Autodesk Inventor part; units mm, degrees
ref_plane "YZ Plane" through (0, 0, 0) normal (1, 0, 0) x (0, 1, 0)
ref_plane "XZ Plane" through (0, 0, 0) normal (0, 1, 0) x (-1, 0, 0)
ref_plane "XY Plane" through (0, 0, 0) normal (0, 0, 1) x (1, 0, 0)
sketch "Sketch1" plane through (0, 0, 0) normal (1, 0, 0) x (0, 1, 0)
  line L0 (112.7241, 89.8734) -> (-26.9759, 89.8734)
  line L1 (-26.9759, 89.8734) -> (-26.9759, -24.4266)
  line L2 (-26.9759, -24.4266) -> (112.7241, -24.4266)
  line L3 (112.7241, -24.4266) -> (112.7241, 89.8734)
  point P0 (0, 0)
  dimension "d0" = 114.3
  dimension "d1" = 139.7
extrude "Extrusion1" add sketch "Sketch1" along normal blind 127
sketch "Sketch2" plane through (0, 112.7241, 89.8734) normal (0, 1, 0) x (1, 0, 0)
  line L0 (0, 0) -> (127, 0)
  line L1 (0, 114.3) -> (127, 114.3)
  line L2 (25.4, 0) -> (127, 0)
  line L3 (127, 0) -> (127, 114.3)
  line L4 (127, 114.3) -> (25.4, 114.3)
  line L5 (25.4, 114.3) -> (25.4, 0)
  line L6 (0, 114.3) -> (0, 0)
  point P0 (0, 89.8734)
  dimension "d4" = 25.4
extrude "Extrusion2" cut sketch "Sketch2" against normal blind 25.4 contours L5 L1 L3 L0
sketch "Sketch4" plane through (0, 87.3241, 89.8734) normal (0, 1, 0) x (1, 0, 0)
  line L0 (38.1, 127) -> (38.1, 0)
  circle A0 centre (76.2, 57.15) radius 44.45
  line L1 (127, 114.3) -> (127, 0)
  line L2 (127, 0) -> (25.4, 0)
  point P0 (0, 89.8734)
  dimension "d15" = 50.8
  dimension "d16" = 57.15
  dimension "d54" = 88.9
extrude "Extrusion4" cut sketch "Sketch4" against normal blind 63.5
fillet "Fillet3" radius 38.1 1 edges at (127, 30.1741, 89.8734)
fillet "Fillet4" radius 38.1 1 edges at (127, 30.1741, -24.4266)
sketch "Sketch9" plane through (25.4, 112.7241, 89.8734) normal (1, 0, 0) x (0, 0, -1)
  line L0 (0, 0) -> (114.3, 0)
  line L1 (0, -25.4) -> (0, 0)
  point P0 (89.8734, -112.7241)
  point P1 (57.15, -12.7)
  dimension "d30" = 12.7
  dimension "d31" = 57.15
hole "Hole1" at (25.4, 100.0241, 32.7234) direction (-1, 0, 0) diameter 8.4328 end through all counterbore diameter 20.6502 counterbore depth 5.969
sketch "Sketch10" plane through (0, -26.9759, -24.4266) normal (0, -1, 0) x (1, 0, 0)
  line L0 (0, 114.3) -> (88.9, 114.3)
  line L1 (25.4, 114.3) -> (127, 114.3)
  line L2 (127, 114.3) -> (127, 0)
  line L3 (127, 0) -> (25.4, 0)
  line L4 (25.4, 0) -> (25.4, 114.3)
  line L5 (0, 114.3) -> (0, 0)
  point P0 (0, 24.4266)
  dimension "d39" = 25.4
  dimension "d42" = 114.3
  dimension "d60" = 101.6
extrude "Extrusion6" cut sketch "Sketch10" against normal blind 25.4
sketch "Sketch11" plane through (25.4, -26.9759, 89.8734) normal (1, 0, 0) x (0, 0, -1)
  line L0 (114.3, 0) -> (0, 0)
  line L1 (114.3, 25.4) -> (114.3, 0)
  point P0 (89.8734, 26.9759)
  point P1 (57.15, 12.7)
  dimension "d43" = 12.7
  dimension "d44" = 57.15
hole "Hole2" at (25.4, -14.2759, 32.7234) direction (-1, 0, 0) diameter 8.4328 end through all counterbore diameter 20.6502 counterbore depth 5.969
sketch "Sketch15" plane through (0, -26.9759, -24.4266) normal (0, 0, -1) x (-1, 0, 0)
  line L0 (-25.4, 114.3) -> (-88.9, 114.3)
  line L1 (-76.2, 114.3) -> (-69.85, 114.3)
  line L2 (-69.85, 114.3) -> (-69.85, 50.8)
  line L3 (-69.85, 50.8) -> (-76.2, 50.8)
  line L4 (-76.2, 50.8) -> (-76.2, 114.3)
  line L5 (-127, 114.3) -> (-127, 0)
  point P0 (0, 26.9759)
  point P1 (-127, 25.4)
  dimension "d55" = 6.35
  dimension "d56" = 50.8
  dimension "d57" = 63.5
extrude "Extrusion8" cut sketch "Sketch15" against normal blind 25.4
properties part number "Cleaning Bottle Holder"
Work out the finished part from the listing and answer in its coordinate system (mm). A direction names the side the tool comes from. Round coordinates to 2 decimals unless told otherwise and drop trailing zeros. Order: outer loops, then holes, each group sorted by start corner. A loop starts at its lowest first (then second) coordinate and runs counter-clockwise, first axis right, second up. Notation, with made-up numbers: M -20,78 L -2,78 A31 ccw -2,109 Z; hole C -4.75,-34 d7. An arc over 180 degrees is marked long. One line per item, written item: value.
Q1. Find section D-D on y = 7. Write down the section's boundary in (x, z), then the cut area to 3 significant figures.
Derived:
outline: M 0,-24.43 L 88.9,-24.43 A38.1 ccw 127,13.67 L 127,51.77 A38.1 ccw 88.9,89.87 L 0,89.87 Z
area: 13,900 mm²
Q2. Determine the mould class of faces 1 (the face through (9.579, 99.839, 36.936)), 2 (the face through (25.4, 89, 32)), 3 (the face through (19.431, -9.8, 32.9)), 4 (the face through (30, 87.324, 32)) for opening direction Y: released by +Y, released by -Y, zero draft, split by the parting line, or undercut.
Derived:
face 1: undercut
face 2: zero draft
face 3: undercut
face 4: released by +Y
Q3. Flat-ended cylindrical pins translate along their axes: pin 1 (14.5 mm diameter, centred on y = 58.5, z = -20, fed in from +X); pin 2 (11 mm diameter, centred on y = 100.02, z = 32.72, fed in from +X); pin 3 (12 mm diameter, centred on y = -12, z = 14, fed in from +X). Find the tip coordinate at first contact, or state that the pin passes through.
Derived:
pin 1: x = 116.35
pin 2: x = 19.43
pin 3: x = 25.4
Q4. Find section C-C on x = 85. Write down the section's boundary in (y, z).
Derived:
outline: M -1.58,-24.43 L 87.32,-24.43 L 87.32,-10.85 L 23.82,-10.85 L 23.82,76.29 L 87.32,76.29 L 87.32,89.87 L -1.58,89.87 Z
Q5. Straight lines are drawn through the part: line 1 (Z direction, x = 15.5, y = -14.5); line 2 (Z direction, x = 80.5, y = 67); line 3 (Y direction, x = 87, z = 19.5). For each, find the intervals that lie inside material, in ascending order.
Derived:
line 1: -24.43 to 28.51, 36.93 to 89.87
line 2: -24.43 to -11.52, 76.96 to 89.87
line 3: -1.58 to 23.82
Q6. Find section A-A on y = 44. Write down the section's boundary in (x, z).
Derived:
outline: M 0,-24.43 L 69.85,-24.43 L 69.85,-11.27 A44.45 cw long 76.2,-11.73 L 76.2,-24.43 L 88.9,-24.43 A38.1 ccw 127,13.67 L 127,51.77 A38.1 ccw 88.9,89.87 L 0,89.87 Z
Q7. For faces 5 (the face through (69.85, 56, -18)), 6 (the face through (22.37, -14.73, 43.04)), 7 (the face through (25.4, -26, 32)), determine the directions among +Z, -Z, +X, -X, +Y, -Y from which every point of the face is accessible in a straight line to the end or side of a thin tool.
Derived:
face 5: -Z, +Y
face 6: +X
face 7: +Z, -Z, +X, -Y
Q8. Find section B-B on z = -5. Write down the section's boundary in (x, y).
Derived:
outline: M 0,-26.98 L 25.4,-26.98 L 25.4,-1.58 L 122.11,-1.58 L 122.11,87.32 L 99.71,87.32 L 99.71,23.82 L 52.69,23.82 L 52.69,87.32 L 25.4,87.32 L 25.4,112.72 L 0,112.72 Z
